Part model, mm, in its own coordinate system. Face numbers are marked on the shaded views. A direction names the side the tool comes from. Round coordinates to 2 decimals unless told otherwise and drop trailing zeros. Order: outer loops, then holes, each group sorted by start corner. A loop starts at its lowest first (then second) coordinate and runs counter-clockwise, first axis right, second up. Notation, with made-up numbers: (57, 23.25) - (100, 23.25) arc R29 cw to (100, 49.25) - close; hole circle Ø9 at (30.25, -12). An arc over 180 degrees is marked (long way). Answer as a JSON object with one key per item and string values.
```python
from build123d import *

# Parameters (mm, degrees)
SKETCH1_W           = 120
SKETCH1_H           = 120
BOSS_EXTRUDE1_DEPTH = 90
FILLET1_R           = 5
SHELL1_T            = -4
CUT_EXTRUDE1_DEPTH  = 30


with BuildPart() as part:
    # Sketch1 → Boss-Extrude1 (new body)
    with BuildSketch(Plane.XY):
        Rectangle(SKETCH1_W, SKETCH1_H)
    extrude(amount=BOSS_EXTRUDE1_DEPTH)

    # Fillet1
    fillet1_edges = [part.edges().sort_by_distance(p)[0] for p in [
        (60, -60, 45),
        (-60, -60, 45),
        (-60, 60, 45),
        (60, 60, 45),
    ]]
    fillet(fillet1_edges, radius=FILLET1_R)

    # Shell1
    shell1_openings = [part.faces().sort_by_distance(p)[0] for p in [
        (0, 0, 90),
    ]]
    offset(amount=SHELL1_T, openings=shell1_openings, kind=Kind.INTERSECTION)

    # Sketch2 → Cut-Extrude1 (cut)
    with BuildSketch(Plane.XY.offset(90)):
        with BuildLine():
            Line((-55, -60), (55, -60))
            ThreePointArc((55, -60), (58.535533906, -58.535533906), (60, -55))
            Line((60, -55), (60, 55))
            ThreePointArc((60, 55), (58.535533906, 58.535533906), (55, 60))
            Line((55, 60), (-55, 60))
            ThreePointArc((-55, 60), (-58.535533906, 58.535533906), (-60, 55))
            Line((-60, 55), (-60, -55))
            ThreePointArc((-60, -55), (-58.535533906, -58.535533906), (-55, -60))
        make_face()
        with BuildLine():
            Line((55, 58), (-55, 58))
            ThreePointArc((-55, 58), (-57.121320344, 57.121320344), (-58, 55))
            Line((-58, 55), (-58, -55))
            ThreePointArc((-58, -55), (-57.121320344, -57.121320344), (-55, -58))
            Line((-55, -58), (55, -58))
            ThreePointArc((55, -58), (57.121320344, -57.121320344), (58, -55))
            Line((58, -55), (58, 55))
            ThreePointArc((58, 55), (57.121320344, 57.121320344), (55, 58))
        make_face(mode=Mode.SUBTRACT)
    extrude(amount=-CUT_EXTRUDE1_DEPTH, mode=Mode.SUBTRACT)


solid = part.part
```
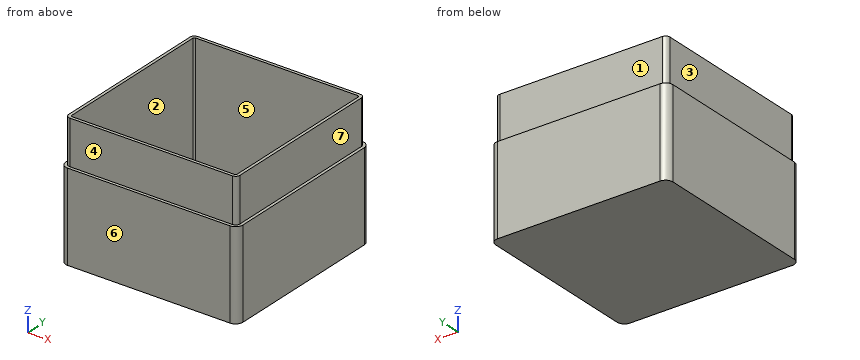
Item 1: Probe L1, parallel to X at y = 3, z = 29; L2, parallel to Y at x = -10, z = 69. List the from-to ranges inside material, lowest first. Write a range as from..to.
Taken from the geometry:
{"L1": "-60..-56, 56..60", "L2": "-58..-56, 56..58"}
Item 2: Drop flat-ended pins along their axis: P1, Ø6, axis at x = -17.5, y = 7.5, coming from the +Z side; P2, Ø1, axis at y = 34, z = 64, coming from the +X side; P3, Ø24, axis at y = 23.5, z = 77.5, coming from the -X side. Give the stop position or say it passes through.
Taken from the geometry:
{"P1": "z = 4", "P2": "x = 58", "P3": "x = -58"}
Item 3: Two-plate mould, pull along X, no slides. Class the marked faces 5, 6 and 7: pulls with the +X half, pulls with the -X half, needs draft (parallel to the pull), parting line crosses it, or undercut.
Taken from the geometry:
{"face 5": "undercut", "face 6": "needs draft", "face 7": "pulls with the +X half"}
Item 4: Tool access for the marked faces 1, 2, 3 and 4: list every direction of +Z, -Z, +X, -X, +Y, -Y with a clear straight run to the whole face (end or side of a thin tool).
Taken from the geometry:
{"face 1": "+Z, +X, -X, +Y", "face 2": "+Z", "face 3": "+Z, -X, +Y, -Y", "face 4": "+Z, +X, -X, -Y"}
Item 5: Cut at B-B (y = 49). Write the cut outline in (x, z).
Taken from the geometry:
{"outline": "(-60, 0) - (60, 0) - (60, 60) - (58, 60) - (58, 90) - (56, 90) - (56, 4) - (-56, 4) - (-56, 90) - (-58, 90) - (-58, 60) - (-60, 60) - close"}
Item 6: Cut at D-D (z = 49.5). Write the cut outline in (x, y), plus the area to 3 significant figures.
Taken from the geometry:
{"outline": "(-60, -55) arc R5 ccw to (-55, -60) - (55, -60) arc R5 ccw to (60, -55) - (60, 55) arc R5 ccw to (55, 60) - (-55, 60) arc R5 ccw to (-60, 55) - close; hole (-56, -55) arc R1 ccw to (-55, -56) - (55, -56) arc R1 ccw to (56, -55) - (56, 55) arc R1 ccw to (55, 56) - (-55, 56) arc R1 ccw to (-56, 55) - close", "area": "1,840 mm2"}
Item 7: Cut at A-A (z = 81). Write the cut outline in (x, y).
Taken from the geometry:
{"outline": "(-58, -55) arc R3 ccw to (-55, -58) - (55, -58) arc R3 ccw to (58, -55) - (58, 55) arc R3 ccw to (55, 58) - (-55, 58) arc R3 ccw to (-58, 55) - close; hole (-56, -55) arc R1 ccw to (-55, -56) - (55, -56) arc R1 ccw to (56, -55) - (56, 55) arc R1 ccw to (55, 56) - (-55, 56) arc R1 ccw to (-56, 55) - close"}
